Check sheet for the modelled part. Datum: model origin and axes. Units: mm. A direction names the side the tool comes from. Round coordinates to 2 decimals unless told otherwise and drop trailing zeros. Loops run counter-clockwise (first coordinate to the right, second up) from the corner with the lowest first, then second, coordinate; pieces in that order, holes last. Notation, with made-up numbers: (42, -28) - (46, -28) arc R26 ccw to (46, -9) - close; hole circle Ø2 at (-27.75, 1.25). An arc over 180 degrees is marked (long way). Answer in a Markdown table with one row per item. Add a question column.
(1) Cross-section at D-D on x = 0. Enter the section's corners in (y, z).
(2) Thickness scan on line 1 along Z through (x, y) = (-11.65, 46.99); line 2 along Z through (x, y) = (-9.25, 38.5). Record the ranges inside material, lowest first.
(3) Cross-section at B-B on x = 9.25. Enter the section's corners in (y, z), then the cut area to 3 significant figures.
(4) Access from +Z, -Z, +X, -X, +Y, -Y to the whole of each face (thin tool, end or side, straight path). Record for faces 1 (the flat face through (5, 31, -11.112)), 2 (the flat face through (5, 31, 12.7)).
(5) Cross-section at A-A on y = 46.99. Enter the section's corners in (x, z), then the cut area to 4 significant figures.
(6) Cross-section at C-C on z = 8.89. Enter the section's corners in (x, y).
(7) Gauge pin test, flat end, axial feed: pin 1 (12.5 mm diameter, centred on x = 0, y = 23.85, fed in from +Z). Record the tip position at first contact, or that the pin passes through.
(8) Mould release check, pull along X, two halves, no side actions. Record for faces 3 (the cylindrical face through (1.035, 15.968, 11.895)), 4 (the flat face through (-11.3, 50.8, -0.1)), 5 (the flat face through (12.7, 25, 0)), 6 (the flat face through (-11.112, 25, 0)): +X half, -X half, draft (parallel to the pull), parting line (faces both ways), or undercut.
from build123d import *

# Parameters (mm, degrees)
SKETCH1_W               = 25.4
SKETCH1_H               = 25.4
SKETCH1_W_2             = 22.225
SKETCH1_H_2             = 22.225
BOSS_EXTRUDE1_DEPTH     = 50.8
CUT_EXTRUDE1_DEPTH      = 59.198711326
CUT_EXTRUDE1_DEPTH_BACK = 59.198711326
SKETCH2_R               = 7.9502
CUT_EXTRUDE2_DEPTH      = 59.198711326
CUT_EXTRUDE2_DEPTH_BACK = 59.198711326
SKETCH3_R               = 1.4732


with BuildPart() as part:
    # Sketch1 → Boss-Extrude1 (new body)
    with BuildSketch(Plane(origin=(0, 0, 0), x_dir=(1, 0, 0), z_dir=(0, 1, 0))):
        Rectangle(SKETCH1_W, SKETCH1_H)
        Rectangle(SKETCH1_W_2, SKETCH1_H_2, mode=Mode.SUBTRACT)
    extrude(amount=BOSS_EXTRUDE1_DEPTH)

    # Sketch2 → Cut-Extrude1 (cut, two sides: drawn at the far end of the back side and taken through both)
    with BuildSketch(Plane.XY.offset(12.7).offset(-CUT_EXTRUDE1_DEPTH_BACK)):
        with Locations(Location((0, 23.8506, 0), (0, 0, 180))):
            Circle(SKETCH2_R)
    extrude(amount=CUT_EXTRUDE1_DEPTH + CUT_EXTRUDE1_DEPTH_BACK, mode=Mode.SUBTRACT)

    # Sketch3 → Cut-Extrude2 (cut, two sides: drawn at the far end of the back side and taken through both)
    with BuildSketch(Plane(origin=(12.7, 0, 0), x_dir=(0, 0, -1), z_dir=(1, 0, 0)).offset(-CUT_EXTRUDE2_DEPTH_BACK)):
        with Locations((-8.89, 46.99)):
            Circle(SKETCH3_R)
        with Locations((8.89, 46.99)):
            Circle(SKETCH3_R)
    extrude(amount=CUT_EXTRUDE2_DEPTH + CUT_EXTRUDE2_DEPTH_BACK, mode=Mode.SUBTRACT)


solid = part.part
Answers:
| question | item | result |
|---|---|---|
| 1 | outline | (0, -12.7) - (15.9, -12.7) - (15.9, -11.11) - (0, -11.11) - close; (0, 11.11) - (15.9, 11.11) - (15.9, 12.7) - (0, 12.7) - close; (31.8, -12.7) - (50.8, -12.7) - (50.8, -11.11) - (31.8, -11.11) - close; (31.8, 11.11) - (50.8, 11.11) - (50.8, 12.7) - (31.8, 12.7) - close |
| 2 | line 1 | z = -12.7 to -10.36, -7.42 to 7.42, 10.36 to 12.7 |
| 2 | line 2 | z = -12.7 to -11.11, 11.11 to 12.7 |
| 3 | outline | (0, -12.7) - (50.8, -12.7) - (50.8, -11.11) - (0, -11.11) - close; (0, 11.11) - (50.8, 11.11) - (50.8, 12.7) - (0, 12.7) - close |
| 3 | area | 161 mm^2 |
| 4 | face 1 | +Y, -Y |
| 4 | face 2 | +Z, +X, -X, +Y, -Y |
| 5 | outline | (-12.7, -12.7) - (12.7, -12.7) - (12.7, -10.36) - (11.11, -10.36) - (11.11, -11.11) - (-11.11, -11.11) - (-11.11, -10.36) - (-12.7, -10.36) - close; (-12.7, -7.42) - (-11.11, -7.42) - (-11.11, 7.42) - (-12.7, 7.42) - close; (-12.7, 10.36) - (-11.11, 10.36) - (-11.11, 11.11) - (11.11, 11.11) - (11.11, 10.36) - (12.7, 10.36) - (12.7, 12.7) - (-12.7, 12.7) - close; (11.11, -7.42) - (12.7, -7.42) - (12.7, 7.42) - (11.11, 7.42) - close |
| 5 | area | 132.5 mm^2 |
| 6 | outline | (-12.7, 0) - (-11.11, 0) - (-11.11, 45.52) - (-12.7, 45.52) - close; (-12.7, 48.46) - (-11.11, 48.46) - (-11.11, 50.8) - (-12.7, 50.8) - close; (11.11, 0) - (12.7, 0) - (12.7, 45.52) - (11.11, 45.52) - close; (11.11, 48.46) - (12.7, 48.46) - (12.7, 50.8) - (11.11, 50.8) - close |
| 7 | pin 1 | passes through |
| 8 | face 3 | undercut |
| 8 | face 4 | draft |
| 8 | face 5 | +X half |
| 8 | face 6 | undercut |
